```python
from build123d import *

# Parameters (mm, degrees)
SKETCH1_W           = 28
SKETCH1_H           = 7.75
BOSS_EXTRUDE1_DEPTH = 1.6
SKETCH2_R           = 1.5
CUT_EXTRUDE1_DEPTH  = 2.6
SKETCH3_R           = 0.55
CUT_EXTRUDE2_DEPTH  = 2.6
FILLET1_R           = 3


with BuildPart() as part:
    # Sketch1 → Boss-Extrude1 (new body)
    with BuildSketch(Plane.XY):
        Rectangle(SKETCH1_W, SKETCH1_H)
    extrude(amount=BOSS_EXTRUDE1_DEPTH)

    # Sketch2 → Cut-Extrude1 (cut, through all)
    with BuildSketch(Plane.XY.offset(1.6)):
        with Locations((-10.05, 0)):
            Circle(SKETCH2_R)
        with Locations((9.95, 0)):
            Circle(SKETCH2_R)
    extrude(amount=-CUT_EXTRUDE1_DEPTH, mode=Mode.SUBTRACT)

    # Sketch3 → Cut-Extrude2 (cut, through all)
    with BuildSketch(Plane.XY.offset(1.6)):
        with Locations((0, -2.475)):
            Circle(SKETCH3_R)
        with Locations((-5.08, -2.475)):
            Circle(SKETCH3_R)
        with Locations((5.08, -2.475)):
            Circle(SKETCH3_R)
    extrude(amount=-CUT_EXTRUDE2_DEPTH, mode=Mode.SUBTRACT)

    # Fillet1
    fillet1_edges = [part.edges().sort_by_distance(p)[0] for p in [
        (14, -3.875, 0.8),
        (-14, -3.875, 0.8),
        (-14, 3.875, 0.8),
        (14, 3.875, 0.8),
    ]]
    fillet(fillet1_edges, radius=FILLET1_R)


solid = part.part
```
For this review, take the finished solid that the model builds, in its own axes (mm). Round coordinates to 2 decimals unless told otherwise and drop trailing zeros. Loops run counter-clockwise (first coordinate to the right, second up) from the corner with the lowest first, then second, coordinate; pieces in that order, holes last.
Q1. Add section B-B on y = 0. Write out the cut boundary in (x, z), plus the area to 3 significant figures.
Result sheet:
outline: (-14, 0) - (-11.55, 0) - (-11.55, 1.6) - (-14, 1.6) - close; (-8.55, 0) - (8.45, 0) - (8.45, 1.6) - (-8.55, 1.6) - close; (11.45, 0) - (14, 0) - (14, 1.6) - (11.45, 1.6) - close
area: 35.2 mm2
Q2. To check wall thickness, follow line 1 along Y through (x, z) = (9.95, 0.85) (3 decimals); line 2 along X through (y, z) = (0.5, 0.6); line 3 along Y through (x, z) = (5.08, 0.85) (3 decimals). State the ranges of each line that lie inside material, in increasing order.
Result sheet:
line 1: y = -3.875 to -1.5, 1.5 to 3.875
line 2: x = -14 to -11.46, -8.64 to 8.54, 11.36 to 14
line 3: y = -3.875 to -3.025, -1.925 to 3.875
Q3. Add section C-C on z = 1.05. Write out the cut boundary in (x, y) (3 decimals), plus the area to 3 significant figures.
Result sheet:
outline: (-14, -0.875) arc R3 ccw to (-11, -3.875) - (11, -3.875) arc R3 ccw to (14, -0.875) - (14, 0.875) arc R3 ccw to (11, 3.875) - (-11, 3.875) arc R3 ccw to (-14, 0.875) - close; hole circle Ø3 at (-10.05, 0); hole circle Ø1.1 at (-5.08, -2.475); hole circle Ø1.1 at (0, -2.475); hole circle Ø1.1 at (5.08, -2.475); hole circle Ø3 at (9.95, 0)
area: 192 mm2
Q4. Mouldability with a two-part tool opening along Y and no side actions: class faces 1 (the face through (0, -3.875, 1)), 2 (the face through (0, 3.875, 1)), 3 (the face through (-0.12, -3.01, 0.81)), 4 (the face through (14, 0, 1)) as +Y half, -Y half, draft (parallel to the pull), parting line (faces both ways), or undercut.
Result sheet:
face 1: -Y half
face 2: +Y half
face 3: undercut
face 4: draft
Q5. Add section A-A on x = 9.95. Write out the cut boundary in (y, z) (3 decimals), plus the area to 3 significant figures.
Result sheet:
outline: (-3.875, 0) - (-1.5, 0) - (-1.5, 1.6) - (-3.875, 1.6) - close; (1.5, 0) - (3.875, 0) - (3.875, 1.6) - (1.5, 1.6) - close
area: 7.60 mm2
Q6. Insertion check: pin 1 Ø2.5 at (x, y) = (9.95, 0) entering from -Z; pin 2 Ø4 at (x, y) = (-10.05, 0) entering from +Z. Each pin has a flat end and moves straight along its axis. Give the tip position at first contact, or say it passes through.
Result sheet:
pin 1: passes through
pin 2: stops at z = 1.6
Q7. Add section D-D on x = -5.08. Write out the cut boundary in (y, z) (3 decimals).
Result sheet:
outline: (-3.875, 0) - (-3.025, 0) - (-3.025, 1.6) - (-3.875, 1.6) - close; (-1.925, 0) - (3.875, 0) - (3.875, 1.6) - (-1.925, 1.6) - close
